from build123d import *

# Parameters (mm, degrees)
CROQUIS1_W              = 47.6
CROQUIS1_H              = 47.6
SALIENTE_EXTRUIR1_DEPTH = 40
CROQUIS3_R              = 35
SALIENTE_EXTRUIR2_DEPTH = 47.6
CROQUIS4_W              = 80
CROQUIS4_H              = 40
CORTAR_EXTRUIR1_DEPTH   = 81.72025768
CROQUIS9_W              = 90
CROQUIS9_H              = 10
SALIENTE_EXTRUIR3_DEPTH = 47.6
CORTAR_EXTRUIR2_START   = -3.8
CROQUIS5_R              = 27.5
CORTAR_EXTRUIR2_DEPTH   = 37
CROQUIS6_W              = 36
CROQUIS6_H              = 30
CORTAR_EXTRUIR3_DEPTH   = 79.685703911
CORTAR_EXTRUIR4_START   = 10
CROQUIS7_R              = 30
CORTAR_EXTRUIR4_DEPTH   = 17
CROQUIS8_R              = 2.5
CORTAR_EXTRUIR5_DEPTH   = 84.065516311
CROQUIS11_R             = 2.5
CORTAR_EXTRUIR7_DEPTH   = 79.685703911
REDONDEO1_R             = 10
CROQUIS10_R             = 20
CORTAR_EXTRUIR6_DEPTH   = 77.751286634
CROQUIS13_R             = 2
CORTAR_EXTRUIR8_DEPTH   = 77.751286634
CROQUIS14_R             = 6
SALIENTE_EXTRUIR4_DEPTH = 1.2
CROQUIS15_R             = 1.5
CORTAR_EXTRUIR9_DEPTH   = 8


with BuildPart() as part:
    # Croquis1 → Saliente-Extruir1 (new body)
    with BuildSketch(Plane.XY):
        Rectangle(CROQUIS1_W, CROQUIS1_H)
    extrude(amount=SALIENTE_EXTRUIR1_DEPTH)

    # Croquis3 → Saliente-Extruir2 (add)
    with BuildSketch(Plane(origin=(0, 23.8, 0), x_dir=(1, 0, 0), z_dir=(0, 1, 0))):
        with Locations((0, 20)):
            Circle(CROQUIS3_R)
    extrude(amount=-SALIENTE_EXTRUIR2_DEPTH)

    # Croquis4 → Cortar-Extruir1 (cut, through all)
    with BuildSketch(Plane(origin=(0, 23.8, 0), x_dir=(1, 0, 0), z_dir=(0, 1, 0))):
        with Locations((0.60144352, 40)):
            Rectangle(CROQUIS4_W, CROQUIS4_H)
    extrude(amount=-CORTAR_EXTRUIR1_DEPTH, mode=Mode.SUBTRACT)

    # Croquis9 → Saliente-Extruir3 (add)
    with BuildSketch(Plane.XZ.offset(23.8)):
        with Locations((0, -15)):
            Rectangle(CROQUIS9_W, CROQUIS9_H)
    extrude(amount=-SALIENTE_EXTRUIR3_DEPTH)

    # Croquis5 → Cortar-Extruir2 (cut)
    with BuildSketch(Plane(origin=(0, 23.8, 0), x_dir=(1, 0, 0), z_dir=(0, 1, 0)).offset(CORTAR_EXTRUIR2_START)):
        with Locations((0, 20)):
            Circle(CROQUIS5_R)
    extrude(amount=-CORTAR_EXTRUIR2_DEPTH, mode=Mode.SUBTRACT)

    # Croquis6 → Cortar-Extruir3 (cut, through all)
    with BuildSketch(Plane.XY.offset(40)):
        Rectangle(CROQUIS6_W, CROQUIS6_H)
    extrude(amount=-CORTAR_EXTRUIR3_DEPTH, mode=Mode.SUBTRACT)

    # Croquis7 → Cortar-Extruir4 (cut)
    with BuildSketch(Plane.XZ.offset(-20).offset(CORTAR_EXTRUIR4_START)):
        with Locations((0, -20)):
            Circle(CROQUIS7_R)
    extrude(amount=CORTAR_EXTRUIR4_DEPTH, mode=Mode.SUBTRACT)

    # Croquis8 → Cortar-Extruir5 (cut, through all)
    with BuildSketch(Plane(origin=(23.8, 0, 0), x_dir=(0, 0, -1), z_dir=(1, 0, 0))):
        with Locations(Location((-35, 19, 0), (0, 0, 90))):
            Circle(CROQUIS8_R)
        with Locations(Location((-20, 19, 0), (0, 0, 90))):
            Circle(CROQUIS8_R)
        with Locations(Location((-20, -19, 0), (0, 0, 90))):
            Circle(CROQUIS8_R)
        with Locations(Location((-35, -19, 0), (0, 0, 90))):
            Circle(CROQUIS8_R)
    extrude(amount=-CORTAR_EXTRUIR5_DEPTH, mode=Mode.SUBTRACT)

    # Croquis11 → Cortar-Extruir7 (cut, through all)
    with BuildSketch(Plane(origin=(0, 0, -20), x_dir=(-1, 0, 0), z_dir=(0, 0, -1))):
        with Locations((39, 14)):
            Circle(CROQUIS11_R)
        with Locations(Location((39, -14, 0), (0, 0, 180))):
            Circle(CROQUIS11_R)
        with Locations((-39, -14)):
            Circle(CROQUIS11_R)
        with Locations(Location((-39, 14, 0), (0, 0, 180))):
            Circle(CROQUIS11_R)
    extrude(amount=-CORTAR_EXTRUIR7_DEPTH, mode=Mode.SUBTRACT)

    # Redondeo1
    redondeo1_edges = [part.edges().sort_by_distance(p)[0] for p in [
        (45, -23.8, -15),
        (-45, 23.8, -15),
        (45, 23.8, -15),
        (-45, -23.8, -15),
    ]]
    fillet(redondeo1_edges, radius=REDONDEO1_R)

    # Croquis10 → Cortar-Extruir6 (cut, through all)
    with BuildSketch(Plane(origin=(0, 23.8, 0), x_dir=(1, 0, 0), z_dir=(0, 1, 0))):
        with Locations((0, 20)):
            Circle(CROQUIS10_R)
    extrude(amount=-CORTAR_EXTRUIR6_DEPTH, mode=Mode.SUBTRACT)

    # Croquis13 → Cortar-Extruir8 (cut, through all)
    with BuildSketch(Plane(origin=(0, 23.8, 0), x_dir=(1, 0, 0), z_dir=(0, 1, 0))):
        with Locations(Location((-14, -12, 0), (0, 0, 270))):
            Circle(CROQUIS13_R)
        with Locations(Location((14, -12, 0), (0, 0, 270))):
            Circle(CROQUIS13_R)
    extrude(amount=-CORTAR_EXTRUIR8_DEPTH, mode=Mode.SUBTRACT)

    # Croquis14 → Saliente-Extruir4 (add)
    with BuildSketch(Plane.XZ.offset(23.8)):
        with Locations(Location((-18.738329701, -1.261670299, 0), (0, 0, 90))):
            Circle(CROQUIS14_R)
        with Locations(Location((18.738329701, -1.261670299, 0), (0, 0, 90))):
            Circle(CROQUIS14_R)
    extrude(amount=SALIENTE_EXTRUIR4_DEPTH)

    # Croquis15 → Cortar-Extruir9 (cut)
    with BuildSketch(Plane.XZ.offset(25)):
        with Locations(Location((18.738329701, -1.261670299, 0), (0, 0, 270))):
            Circle(CROQUIS15_R)
        with Locations(Location((-18.738329701, -1.261670299, 0), (0, 0, 270))):
            Circle(CROQUIS15_R)
    extrude(amount=-CORTAR_EXTRUIR9_DEPTH, mode=Mode.SUBTRACT)


solid = part.part
Geometry: final body of the model. Coordinates: model frame, mm. A direction names the side the tool comes from. Give positions to 0.01 mm unless a question says otherwise; leave off trailing zeros. Order: outer loops, then holes, each group sorted by start corner. A loop starts at its lowest first (then second) coordinate and runs counter-clockwise, first axis right, second up. Notation, with made-up numbers: (48, 65.25) -> (73, 65.25) arc R17 ccw to (73, 90.25) -> close; hole circle Ø11 at (70, 65.5). An arc over 180 degrees is marked (long way). Put each result on its own line as item: value.
Q1. Section D-D, the plane x = 14. Return loops of the section in (y, z), then the cut area to 3 significant figures.
Here are the results:
outline: (-25, -4.94) -> (-23.8, -4.94) -> (-23.8, -5.72) -> (-17, -5.72) -> (-17, 3.67) -> (-15, 3.67) -> (-15, 10) -> (-23.8, 10) -> (-23.8, 2.42) -> (-25, 2.42) -> close; (-23.8, 14) -> (-15, 14) -> (-15, 40) -> (-23.8, 40) -> close; (15, 3.67) -> (20, 3.67) -> (20, -5.72) -> (23.8, -5.72) -> (23.8, 10) -> (15, 10) -> close; (15, 14) -> (23.8, 14) -> (23.8, 40) -> (15, 40) -> close; hole circle Ø5 at (-19, 20); hole circle Ø5 at (-19, 35); hole circle Ø5 at (19, 20); hole circle Ø5 at (19, 35)
area: 599 mm^2
Q2. Section C-C, the plane y = 0.5. Return loops of the section in (x, z).
Here are the results:
outline: (-45, -20) -> (-30, -20) arc R30 cw to (-18, 4) -> (-18, 40) -> (-23.8, 40) -> (-23.8, 5.66) arc R35 ccw to (-33.54, -10) -> (-45, -10) -> close; (18, 4) arc R30 cw to (30, -20) -> (45, -20) -> (45, -10) -> (33.54, -10) arc R35 ccw to (23.8, 5.66) -> (23.8, 40) -> (18, 40) -> close
Q3. Section B-B, the plane x = 4. Return loops of the section in (y, z), then the cut area to 3 significant figures.
Here are the results:
outline: (-23.8, -0.4) -> (-17, -0.4) -> (-17, 7.21) -> (-15, 7.21) -> (-15, 40) -> (-23.8, 40) -> close; (15, 7.21) -> (20, 7.21) -> (20, -0.4) -> (23.8, -0.4) -> (23.8, 40) -> (15, 40) -> close; hole circle Ø5 at (-19, 20); hole circle Ø5 at (-19, 35); hole circle Ø5 at (19, 20); hole circle Ø5 at (19, 35)
area: 579 mm^2
Q4. Reachability of faces 4 (the face through (0, -15, 21)), 5 (the face through (-39, 0, -10)), 6 (the face through (-25, 10, -8)) from +Z, -Z, +X, -X, +Y, -Y: full face, straight path, thin tool, end or side. Return the list, or none.
Here are the results:
face 4: +Z, -Z
face 5: +Z, -X, +Y, -Y
face 6: -Z
Q5. Material intervals for L1, parallel to X at y = 18, z = 12; L2, parallel to X at y = 13.5, z = -15; L3, parallel to X at y = 12, z = 27, sorted ascending.
Here are the results:
L1: x = -23.8 to -16, -12 to 12, 16 to 23.8
L2: x = -45 to -41.45, -36.55 to -27.04, 27.04 to 36.55, 41.45 to 45
L3: x = -23.8 to -18, 18 to 23.8
Q6. Pin query (flat end, axial travel): pin 1 (0.8 mm diameter, centred on x = 19.5, z = -1, fed in from -Y); pin 2 (6 mm diameter, centred on y = 19, z = 20, fed in from -X); pin 3 (4 mm diameter, centred on x = 20.5, y = 3.5, fed in from -Z). Return the tip coordinate at first contact, or that it passes through.
Here are the results:
pin 1: stops at y = -17
pin 2: stops at x = -23.8
pin 3: stops at z = -0.16
Q7. Section A-A, the plane z = 20. Return loops of the section in (x, y).
Here are the results:
outline: (-23.8, -23.8) -> (23.8, -23.8) -> (23.8, -21.5) -> (-23.8, -21.5) -> close; (-23.8, -16.5) -> (23.8, -16.5) -> (23.8, 16.5) -> (-23.8, 16.5) -> close; (-23.8, 21.5) -> (23.8, 21.5) -> (23.8, 23.8) -> (-23.8, 23.8) -> close; hole (-18, -15) -> (18, -15) -> (18, 15) -> (-18, 15) -> close
Q8. Draft query along Y for faces 1 (the face through (41.99, 20.95, -14.93)), 2 (the face through (0.33, 17.16, 21.69)), 3 (the face through (24.596, -24.392, -2.562)). Return one class per face: released by +Y, released by -Y, zero draft, split by the parting line, or undercut.
Here are the results:
face 1: released by +Y
face 2: undercut
face 3: zero draft
